```python
from build123d import *

# Parameters (mm, degrees)
SKETCH2_W           = 10
SKETCH2_H           = 10
SKETCH2_W_2         = 6.4
SKETCH2_H_2         = 6.4
SKETCH2_R           = 2
BOSS_EXTRUDE1_DEPTH = 4
SKETCH2_3_W         = 10
SKETCH2_3_H         = 10
SKETCH2_3_W_2       = 6.4
SKETCH2_3_H_2       = 6.4
BOSS_EXTRUDE2_DEPTH = 12
SKETCH2_4_W         = 10
SKETCH2_4_H         = 10
BOSS_EXTRUDE3_DEPTH = 12
SKETCH3_R           = 1.25
CUT_EXTRUDE1_DEPTH  = 12
SKETCH4_R           = 1.1
CUT_EXTRUDE2_DEPTH  = 10
FILLET1_R           = 2
SKETCH5_W           = 7
SKETCH5_H           = 7
CUT_EXTRUDE3_DEPTH  = 14


with BuildPart() as part:
    # Sketch2 → Boss-Extrude1 (new body)
    # profile 1 of 2: a face of its own
    with BuildSketch(Plane(origin=(0, 0, 0), x_dir=(1, 0, 0), z_dir=(0, 1, 0))):
        Rectangle(SKETCH2_W, SKETCH2_H)
        Rectangle(SKETCH2_W_2, SKETCH2_H_2, mode=Mode.SUBTRACT)
    # profile 2 of 2: a face of its own
    with BuildSketch(Plane(origin=(0, 0, 0), x_dir=(1, 0, 0), z_dir=(0, 1, 0))):
        Rectangle(SKETCH2_W_2, SKETCH2_H_2)
        with Locations(Location((0, 0, 0), (0, 0, 270))):
            Circle(SKETCH2_R, mode=Mode.SUBTRACT)
    extrude(amount=BOSS_EXTRUDE1_DEPTH)

    # Sketch2_3 → Boss-Extrude2 (add)
    with BuildSketch(Plane(origin=(0, 0, 0), x_dir=(1, 0, 0), z_dir=(0, 1, 0))):
        Rectangle(SKETCH2_3_W, SKETCH2_3_H)
        Rectangle(SKETCH2_3_W_2, SKETCH2_3_H_2, mode=Mode.SUBTRACT)
    extrude(amount=BOSS_EXTRUDE2_DEPTH)

    # Sketch2_4 → Boss-Extrude3 (add)
    with BuildSketch(Plane(origin=(0, 0, 0), x_dir=(1, 0, 0), z_dir=(0, 1, 0))):
        with Locations((10, 0)):
            Rectangle(SKETCH2_4_W, SKETCH2_4_H)
    extrude(amount=BOSS_EXTRUDE3_DEPTH)

    # Sketch3 → Cut-Extrude1 (cut)
    with BuildSketch(Plane.XY.offset(5)):
        with Locations((10, 6)):
            Circle(SKETCH3_R)
    extrude(amount=-CUT_EXTRUDE1_DEPTH, mode=Mode.SUBTRACT)

    # Sketch4 → Cut-Extrude2 (cut)
    with BuildSketch(Plane(origin=(15, 0, 0), x_dir=(0, 0, -1), z_dir=(1, 0, 0))):
        with Locations((0, 9)):
            Circle(SKETCH4_R)
        with Locations(Location((0, 3, 0), (0, 0, 180))):
            Circle(SKETCH4_R)
    extrude(amount=-CUT_EXTRUDE2_DEPTH, mode=Mode.SUBTRACT)

    # Fillet1
    fillet1_edges = [part.edges().sort_by_distance(p)[0] for p in [
        (-5, 6, -5),
        (-5, 6, 5),
        (15, 6, 5),
        (15, 6, -5),
    ]]
    fillet(fillet1_edges, radius=FILLET1_R)

    # Sketch5 → Cut-Extrude3 (cut)
    with BuildSketch(Plane(origin=(0, 12, 0), x_dir=(1, 0, 0), z_dir=(0, 1, 0))):
        with Locations((9.5, 0)):
            Rectangle(SKETCH5_W, SKETCH5_H)
    extrude(amount=-CUT_EXTRUDE3_DEPTH, mode=Mode.SUBTRACT)


solid = part.part
```
Geometry check sheet. Reference: the model listing, model coordinates, mm. A direction names the side the tool comes from. Give positions to 0.01 mm unless a question says otherwise; leave off trailing zeros. Loops run counter-clockwise (first coordinate to the right, second up) from the corner with the lowest first, then second, coordinate; pieces in that order, holes last. Notation, with made-up numbers: M 50,24 L 55,24 A20 ccw 55,41 Z; hole C -12,10 d6. An arc over 180 degrees is marked long. Write item = value, one per line.
(1) Sectioned sample at A-A, the plane y = 6. Record the cut outline in (x, z).
Answer below:
outline = M -5,-3 A2 ccw -3,-5 L 8.75,-5 L 8.75,-3.5 L 6,-3.5 L 6,3.5 L 8.75,3.5 L 8.75,5 L -3,5 A2 ccw -5,3 Z; M 11.25,-5 L 13,-5 A2 ccw 15,-3 L 15,3 A2 ccw 13,5 L 11.25,5 L 11.25,3.5 L 13,3.5 L 13,-3.5 L 11.25,-3.5 Z; hole M -3.2,-3.2 L 3.2,-3.2 L 3.2,3.2 L -3.2,3.2 Z
(2) Release check for a two-part mould opening along Z. For faces 5 (the face through (5, 6, -5)), 6 (the face through (-5, 6, 0)), 7 (the face through (9, 7, -3.5)) record: released by +Z, released by -Z, zero draft, split by the parting line, or undercut.
Answer below:
face_5 = released by -Z
face_6 = zero draft
face_7 = undercut
(3) Gauge pin test, flat end, axial feed: pin 1 Ø0.7 at (y, z) = (3, -0.5) entering from +X. Record the tip position at first contact, or that the pin passes through.
Answer below:
pin_1 = 5
(4) Sectioned sample at B-B, the plane x = 0. Record the cut outline in (y, z).
Answer below:
outline = M 0,-5 L 12,-5 L 12,-3.2 L 4,-3.2 L 4,-2 L 0,-2 Z; M 0,2 L 4,2 L 4,3.2 L 12,3.2 L 12,5 L 0,5 Z
(5) Material ranges on line 1 (Y direction, x = 5.75, z = 0); line 2 (X direction, y = 4.5, z = -2.5); line 3 (Z direction, x = 11.75, y = 2.5), recorded low to high. Write a range as [from, to].
Answer below:
line_1 = [0, 1.9], [4.1, 7.9], [10.1, 12]
line_2 = [-5, -3.2], [3.2, 6], [13, 15]
line_3 = [-5, -3.5], [3.5, 5]
(6) Tool access check on faces 1 (the face through (14.014, 7.926, 0.238)), 2 (the face through (-2.2, 4, 0)), 3 (the face through (15, 6, 0)), 4 (the face through (13, 6, 0)). Record the directions out of +Z, -Z, +X, -X, +Y, -Y that give a thin tool (end or side, any length) a straight path to the whole face; none if there is none.
Answer below:
face_1 = +X
face_2 = +Y
face_3 = +Z, -Z, +X, +Y, -Y
face_4 = +Y, -Y
(7) Sectioned sample at C-C, the plane z = 0. State how many separate pieces and enclosed holes the cut face has, plus the area to 3 significant figures.
Answer below:
separate_pieces = 5
enclosed_holes = 0
area = 75.6 mm2
(8) Sectioned sample at D-D, the plane y = 3. Record the cut outline in (x, z).
Answer below:
outline = M -5,-3 A2 ccw -3,-5 L 13,-5 A2 ccw 15,-3 L 15,-1.1 L 13,-1.1 L 13,-3.5 L 6,-3.5 L 6,-1.1 L 5,-1.1 L 5,1.1 L 6,1.1 L 6,3.5 L 13,3.5 L 13,1.1 L 15,1.1 L 15,3 A2 ccw 13,5 L -3,5 A2 ccw -5,3 Z; hole C 0,0 d4
